Input: part model. Units: mm. Frame: model coordinates. Face numbers are marked on the shaded views. A direction names the side the tool comes from. Coordinates: 2 decimals unless noted, no trailing zeros. Order: outer loops, then holes, each group sorted by start corner. A loop starts at its lowest first (then second) coordinate and runs counter-clockwise, first axis right, second up. Notation, with made-up numbers: M -3.5,10.25 L 44.5,10.25 A24 ccw 44.5,34.25 Z; hole C -16,6 d5. An arc over 180 degrees is marked long. Answer in a Markdown table with one row per item.
from build123d import *

# Parameters (mm, degrees)
SKETCH1_W           = 25.4
SKETCH1_H           = 25.4
BOSS_EXTRUDE1_DEPTH = 25.4
SKETCH2_R           = 3.175
CUT_EXTRUDE1_DEPTH  = 12.7
SKETCH3_R           = 3.175
CUT_EXTRUDE2_DEPTH  = 12.7


with BuildPart() as part:
    # Sketch1 → Boss-Extrude1 (new body)
    with BuildSketch(Plane.XY):
        Rectangle(SKETCH1_W, SKETCH1_H)
    extrude(amount=BOSS_EXTRUDE1_DEPTH)

    # Sketch2 → Cut-Extrude1 (cut)
    with BuildSketch(Plane.XY.offset(25.4)):
        Circle(SKETCH2_R)
    extrude(amount=-CUT_EXTRUDE1_DEPTH, mode=Mode.SUBTRACT)

    # Sketch3 → Cut-Extrude2 (cut)
    with BuildSketch(Plane(origin=(0, 12.7, 0), x_dir=(1, 0, 0), z_dir=(0, 1, 0))):
        with Locations((0, -12.7)):
            Circle(SKETCH3_R)
    extrude(amount=-CUT_EXTRUDE2_DEPTH, mode=Mode.SUBTRACT)


solid = part.part
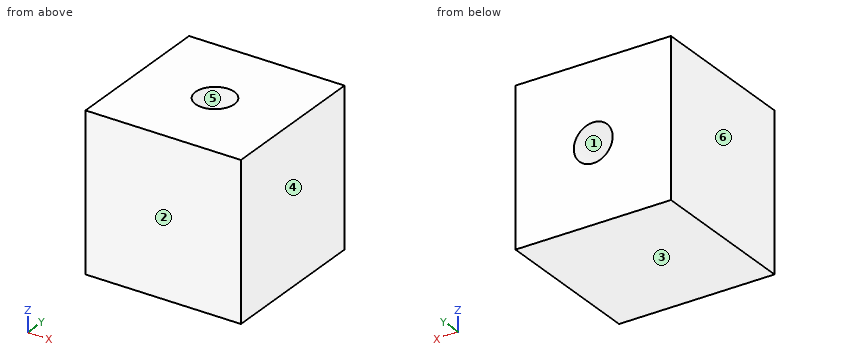
1) Cut plane A-A, the plane x = 0. Output: boundary loops of the cut face in (y, z) (3 decimals).
Resolved:
| item | result |
|---|---|
| outline | M -12.7,0 L 12.7,0 L 12.7,9.525 L 0,9.525 L 0,12.7 L -3.175,12.7 L -3.175,25.4 L -12.7,25.4 Z; M 3.175,15.875 L 12.7,15.875 L 12.7,25.4 L 3.175,25.4 Z |
2) Cut plane C-C, the plane z = 22. Output: boundary loops of the cut face in (x, y) (3 decimals).
Resolved:
| item | result |
|---|---|
| outline | M -12.7,-12.7 L 12.7,-12.7 L 12.7,12.7 L -12.7,12.7 Z; hole C 0,0 d6.35 |
3) Mould query, pull axis X, two halves, no side actions, for the marked faces 3, 4, 5 and 6. Classes: +X half, -X half, draft (parallel to the pull), parting line (faces both ways), or undercut.
Resolved:
| item | result |
|---|---|
| face 3 | draft |
| face 4 | +X half |
| face 5 | undercut |
| face 6 | -X half |
4) Cut plane D-D, the plane z = 12. Output: boundary loops of the cut face in (x, y), and give its area (4 significant figures).
Resolved:
| item | result |
|---|---|
| outline | M -12.7,-12.7 L 12.7,-12.7 L 12.7,12.7 L 3.1,12.7 L 3.1,0 L -3.1,0 L -3.1,12.7 L -12.7,12.7 Z |
| area | 566.5 mm2 |
5) Contact query for a flat-ended pin moving along its axis: pin 1 (5 mm diameter, centred on x = 0, y = 0, fed in from +Z). Output: stop coordinate, or through.
Resolved:
| item | result |
|---|---|
| pin 1 | stops at z = 12.7 |
6) Reachability of the marked faces 1 and 2 from +Z, -Z, +X, -X, +Y, -Y: full face, straight path, thin tool, end or side. Return the list, or none.
Resolved:
| item | result |
|---|---|
| face 1 | +Y |
| face 2 | +Z, -Z, +X, -X, -Y |
7) Material intervals for probe 1 along Z at (x, y) = (0, 5.25) (3 decimals); probe 2 along X at (y, z) = (4.25, 12.7) (3 decimals); probe 3 along Y at (x, z) = (-1.5, 12), sorted ascending.
Resolved:
| item | result |
|---|---|
| probe 1 | z = 0 to 9.525, 15.875 to 25.4 |
| probe 2 | x = -12.7 to -3.175, 3.175 to 12.7 |
| probe 3 | y = -12.7 to 0 |
8) Cut plane B-B, the plane y = 8.5. Output: boundary loops of the cut face in (x, z) (3 decimals), and give its area (3 significant figures).
Resolved:
| item | result |
|---|---|
| outline | M -12.7,0 L 12.7,0 L 12.7,25.4 L -12.7,25.4 Z; hole C 0,12.7 d6.35 |
| area | 613 mm2 |
